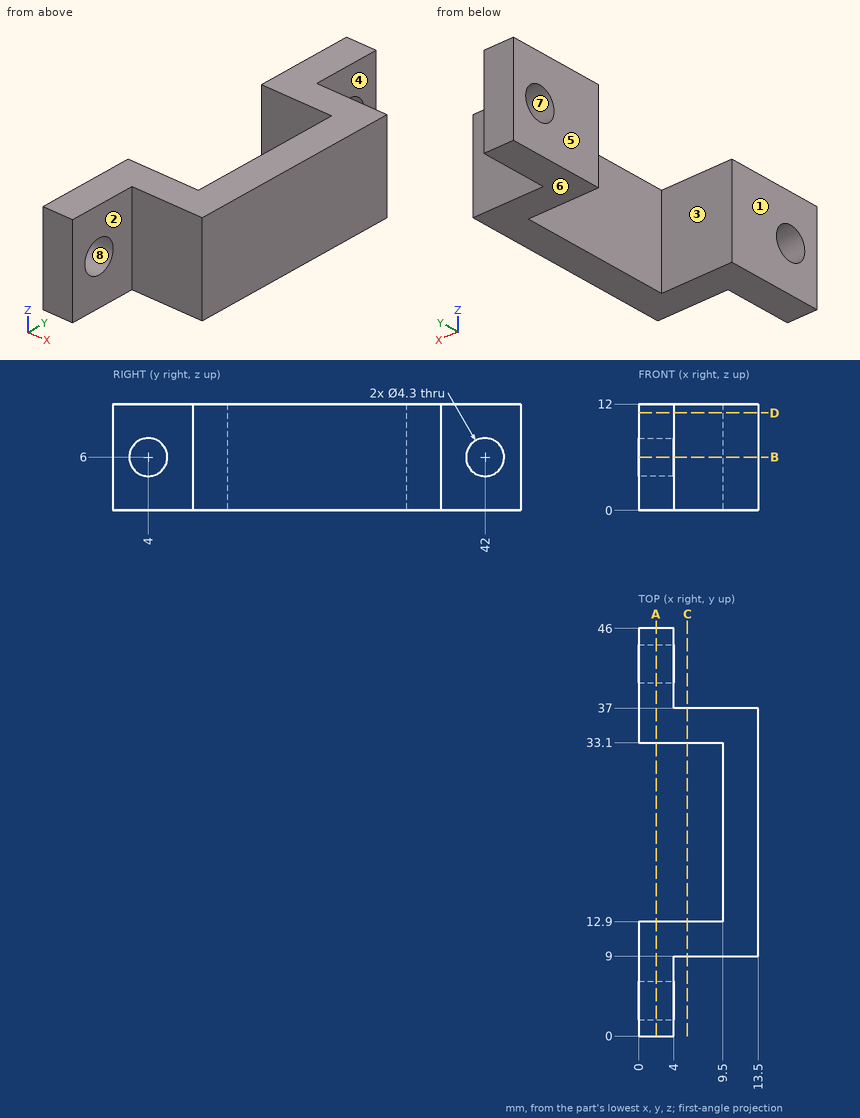
The figure shows three views and two pictorial views of one solid part (mm, origin at its lowest corner). Answer the questions. A direction names the side the tool comes from. Coordinates: 2 decimals unless noted, no trailing zeros. Loops run counter-clockwise (first coordinate to the right, second up) from the corner with the lowest first, then second, coordinate; pieces in that order, holes last. Notation, with made-up numbers: (0.5, 23.5) -> (8.5, 23.5) arc R26 cw to (8.5, 57.5) -> close; hole circle Ø4 at (-24.5, -24). An arc over 180 degrees is marked (long way). Write item = value, one per line. Start each with the question number.
1) A cutting plane is placed at A-A (x = 2). Give the vertices of the cut face in (y, z).
2) A cutting plane is placed at B-B (z = 6). Give the vertices of the cut face in (x, y).
3) A cutting plane is placed at D-D (z = 11). Give the vertices of the cut face in (x, y).
4) A cutting plane is placed at C-C (x = 5.5). Give the vertices of the cut face in (y, z).
5) The mould has two halves that part along Z. Classify the marked faces 5, 6, 7 and 8: released by +Z, released by -Z, zero draft, split by the parting line, or undercut.
6) Given pin 1 Ø4 at (x, z) = (4.5, 8) entering from -Y; pin 2 Ø5 at (x, z) = (7, 4) entering from -Y; pin 3 Ø2.5 at (y, z) = (41, 5.5) entering from +X, each flat-ended and moving along its own axis, determine where each tip first touches the part or whether it passes through.
7) A tool of negligible diameter and unlimited length cuts with its end or side. For the marked faces 1, 2, 3 and 4, from which of +Z, -Z, +X, -X, +Y, -Y can it reach the whole face along a straight path? Write none if from no direction.
8) Straight lines are drawn through the part: line 1 (Y direction, x = 1.1, z = 6); line 2 (Y direction, x = 4.5, z = 6); line 3 (Y direction, x = 11, z = 7.75). For each, find the intervals that lie inside material, in ascending order. Write a range as from..to.
Responses:
q1.outline = (0, 0) -> (12.9, 0) -> (12.9, 12) -> (0, 12) -> close; (33.1, 0) -> (46, 0) -> (46, 12) -> (33.1, 12) -> close; hole circle Ø4.3 at (4, 6); hole circle Ø4.3 at (42, 6)
q2.outline = (0, 0) -> (4, 0) -> (4, 1.85) -> (0, 1.85) -> close; (0, 6.15) -> (4, 6.15) -> (4, 9) -> (13.5, 9) -> (13.5, 37) -> (4, 37) -> (4, 39.85) -> (0, 39.85) -> (0, 33.1) -> (9.5, 33.1) -> (9.5, 12.9) -> (0, 12.9) -> close; (0, 44.15) -> (4, 44.15) -> (4, 46) -> (0, 46) -> close
q3.outline = (0, 0) -> (4, 0) -> (4, 9) -> (13.5, 9) -> (13.5, 37) -> (4, 37) -> (4, 46) -> (0, 46) -> (0, 33.1) -> (9.5, 33.1) -> (9.5, 12.9) -> (0, 12.9) -> close
q4.outline = (9, 0) -> (12.9, 0) -> (12.9, 12) -> (9, 12) -> close; (33.1, 0) -> (37, 0) -> (37, 12) -> (33.1, 12) -> close
q5.face_5 = zero draft
q5.face_6 = released by -Z
q5.face_7 = undercut
q5.face_8 = undercut
q6.pin_1 = 0
q6.pin_2 = 9
q6.pin_3 = 4
q7.face_1 = +Z, -Z, -X, +Y, -Y
q7.face_2 = +Z, -Z, +X, -Y
q7.face_3 = +Z, -Z, -X
q7.face_4 = +Z, -Z, +X, +Y
q8.line_1 = 0..1.85, 6.15..12.9, 33.1..39.85, 44.15..46
q8.line_2 = 9..12.9, 33.1..37
q8.line_3 = 9..37
